Input: part model. Units: mm. Frame: model coordinates. Face numbers are marked on the shaded views. A direction names the side the tool comes from. Round coordinates to 2 decimals unless told otherwise and drop trailing zeros. Order: outer loops, then holes, each group sorted by start corner. A loop starts at its lowest first (then second) coordinate and runs counter-clockwise, first axis right, second up. Notation, with made-up numbers: M 23.25,-28 L 31.25,-28 A11 ccw 31.25,-15 Z; hole C 87,85.25 d6. An arc over 180 degrees is marked long. One line per question, with ' | ' between items.
```python
from build123d import *

# Parameters (mm, degrees)
SKETCH1_R           = 2.025
SKETCH1_R_2         = 3
BOSS_EXTRUDE1_DEPTH = 4
SKETCH2_R           = 10
SKETCH2_R_2         = 7
BOSS_EXTRUDE2_DEPTH = 1
FILLET1_R           = 2


with BuildPart() as part:
    # Sketch1 → Boss-Extrude1 (new body)
    with BuildSketch(Plane(origin=(0, 0, 0), x_dir=(1, 0, 0), z_dir=(0, 1, 0))):
        with BuildLine():
            Line((2.27183836, -8.894641378), (21.255729613, -19.713837864))
            ThreePointArc((21.255729613, -19.713837864), (26.55816164, -19.090358622), (28.724166028, -23.970208697))
            Line((28.724166028, -23.970208697), (33.88183836, -26.909641378))
            ThreePointArc((33.88183836, -26.909641378), (38.370892813, -26.890805018), (40.61, -23))
            Line((40.61, -23), (40.61, 23))
            ThreePointArc((40.61, 23), (38.370892813, 26.890805018), (33.88183836, 26.909641378))
            Line((33.88183836, 26.909641378), (28.724166028, 23.970208697))
            ThreePointArc((28.724166028, 23.970208697), (26.55816164, 19.090358622), (21.255729613, 19.713837864))
            Line((21.255729613, 19.713837864), (2.27183836, 8.894641378))
            ThreePointArc((2.27183836, 8.894641378), (0.609194982, 7.245892813), (0, 4.985))
            Line((0, 4.985), (0, -4.985))
            ThreePointArc((0, -4.985), (0.609194982, -7.245892813), (2.27183836, -8.894641378))
        make_face()
        with Locations((36.11, -23)):
            Circle(SKETCH1_R, mode=Mode.SUBTRACT)
        with Locations((36.11, 23)):
            Circle(SKETCH1_R, mode=Mode.SUBTRACT)
        with Locations((4.5, 4.985)):
            Circle(SKETCH1_R, mode=Mode.SUBTRACT)
        with Locations((4.5, -4.985)):
            Circle(SKETCH1_R, mode=Mode.SUBTRACT)
        with Locations((24.33, 0)):
            Circle(SKETCH1_R_2, mode=Mode.SUBTRACT)
    extrude(amount=BOSS_EXTRUDE1_DEPTH)

    # Sketch2 → Boss-Extrude2 (add)
    with BuildSketch(Plane(origin=(0, 4, 0), x_dir=(1, 0, 0), z_dir=(0, 1, 0))):
        with Locations((24.33, 0)):
            Circle(SKETCH2_R)
        with Locations((24.33, 0)):
            Circle(SKETCH2_R_2, mode=Mode.SUBTRACT)
    extrude(amount=BOSS_EXTRUDE2_DEPTH)

    # Fillet1
    fillet1_edges = [part.edges().sort_by_distance(p)[0] for p in [
        (21.255729613, 2, -19.713837864),
        (28.724166028, 2, -23.970208697),
        (28.724166028, 2, 23.970208697),
        (21.255729613, 2, 19.713837864),
    ]]
    fillet(fillet1_edges, radius=FILLET1_R)


solid = part.part
```
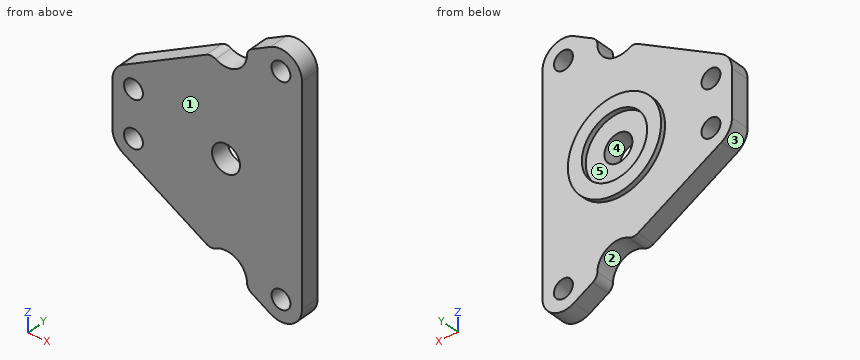
Item 1: Section query C-C, the plane x = 4.5. Return loops of the section in (y, z), plus the area to 3 significant figures.
Report:
outline: M 0,-10.16 L 4,-10.16 L 4,-7.01 L 0,-7.01 Z; M 0,-2.96 L 4,-2.96 L 4,2.96 L 0,2.96 Z; M 0,7.01 L 4,7.01 L 4,10.16 L 0,10.16 Z | area: 48.9 mm²
Item 2: Line query: line 1 along Z through (x, y) = (36.11, 2.8) (3 decimals); line 2 along X through (y, z) = (1.3, -23) (3 decimals); line 3 along Z through (x, y) = (24.33, 2.7). Output: solid intervals per line, ascending. Write a range as from..to.
Report:
line 1: -27.5..-25.025, -20.975..20.975, 25.025..27.5 | line 2: 28.833..34.085, 38.135..40.61 | line 3: -18.5..-3, 3..18.5
Item 3: Mould query, pull axis X, two halves, no side actions, for the marked faces 1, 2 and 3. Classes: +X half, -X half, draft (parallel to the pull), parting line (faces both ways), or undercut.
Report:
face 1: draft | face 2: undercut | face 3: -X half
Item 4: Section query A-A, the plane x = 24.33. Return loops of the section in (y, z).
Report:
outline: M 0,-18.5 L 4,-18.5 L 4,-10 L 5,-10 L 5,-7 L 4,-7 L 4,-3 L 0,-3 Z; M 0,3 L 4,3 L 4,7 L 5,7 L 5,10 L 4,10 L 4,18.5 L 0,18.5 Z
Item 5: Section query D-D, the plane y = 3.25. Return loops of the section in (x, z) (3 decimals).
Report:
outline: M 0,-4.985 A4.5 ccw 2.272,-8.895 L 20.142,-19.079 A2 ccw 22.116,-19.082 A4.5 cw 28.829,-22.908 A2 ccw 29.838,-24.605 L 33.882,-26.91 A4.5 ccw 40.61,-23 L 40.61,23 A4.5 ccw 33.882,26.91 L 29.838,24.605 A2 ccw 28.829,22.908 A4.5 cw 22.116,19.082 A2 ccw 20.142,19.079 L 2.272,8.895 A4.5 ccw 0,4.985 Z; hole C 4.5,-4.985 d4.05; hole C 4.5,4.985 d4.05; hole C 24.33,0 d6; hole C 36.11,-23 d4.05; hole C 36.11,23 d4.05
Item 6: First-contact query: pin 1 (5 mm diameter, centred on x = 13.5, z = -9.5, fed in from +Y); pin 2 (3 mm diameter, centred on x = 8.5, y = 4, fed in from -Z). Flat tips, straight axial feed; report the tip coordinate or a pass-through.
Report:
pin 1: y = 4 | pin 2: z = -13.3
Item 7: Access query for the marked faces 4 and 5. Directions: +Z, -Z, +X, -X, +Y, -Y. A direction counts if a zero-diameter tool reaches every point of the face in a straight line with its end or side. Return the directions, or none.
Report:
face 4: +Y, -Y | face 5: +Y
Item 8: Section query B-B, the plane z = 0. Return loops of the section in (x, y), plus the area to 3 significant figures.
Report:
outline: M 0,0 L 21.33,0 L 21.33,4 L 17.33,4 L 17.33,5 L 14.33,5 L 14.33,4 L 0,4 Z; M 27.33,0 L 40.61,0 L 40.61,4 L 34.33,4 L 34.33,5 L 31.33,5 L 31.33,4 L 27.33,4 Z | area: 144 mm²
